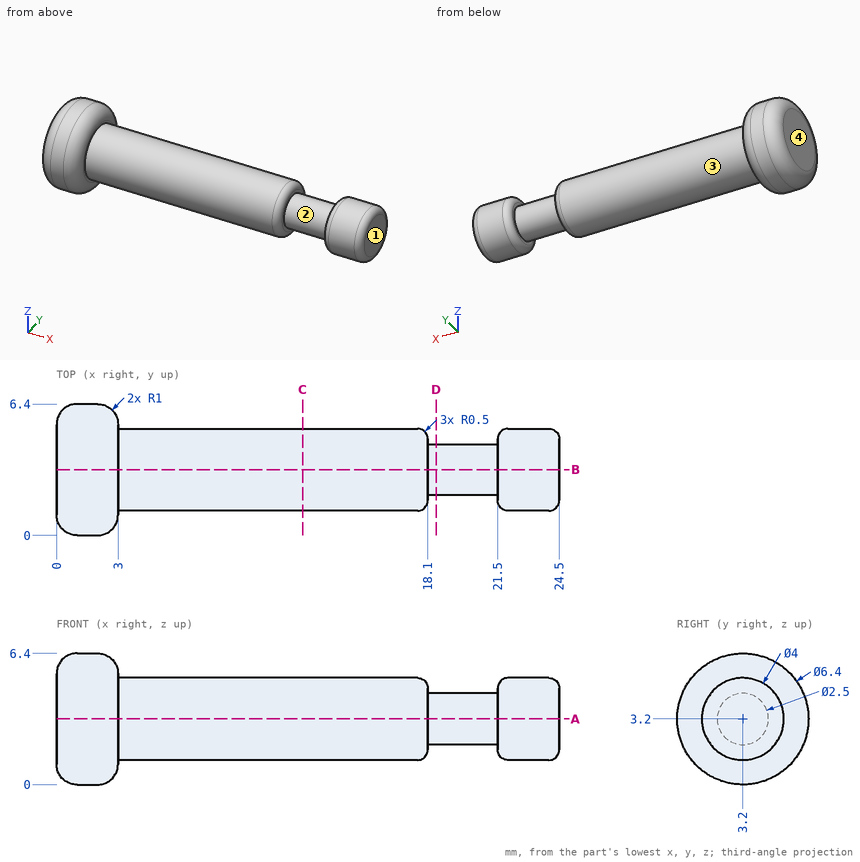
Geometry: see drawing. Coordinates: mm, zero at the bounding-box minimum. Give positions to 0.01 mm unless a question says otherwise; leave off trailing zeros. Order: outer loops, then holes, each group sorted by start corner. A loop starts at its lowest first (then second) coordinate and runs counter-clockwise, first axis right, second up. Notation, with made-up numbers: (86, 39.25) -> (130, 39.25) arc R18 ccw to (130, 64.25) -> close; hole circle Ø7 at (16, -10). An arc over 180 degrees is marked (long way). Write each question's results on one line, items separated by ' | '.
1) Cut plane D-D (x = 18.5). Output: boundary loops of the cut face in (y, z).
Geometry says:
outline: circle Ø2.5 at (3.2, 3.2)
2) Cut plane C-C (x = 12). Output: boundary loops of the cut face in (y, z), and give its area (3 significant figures).
Geometry says:
outline: circle Ø4 at (3.2, 3.2) | area: 12.6 mm²
3) First-contact query: pin 1 Ø3 at (x, y) = (19, 1.5) entering from +Z; pin 2 Ø3 at (x, z) = (17, 4) entering from -Y. Flat tips, straight axial feed; report the tip coordinate or a pass-through.
Geometry says:
pin 1: stops at z = 4.99 | pin 2: stops at y = 1.2
4) Line query: line 1 along X through (y, z) = (2.75, 5.25); line 2 along X through (y, z) = (3.5, 5); line 3 along Z through (x, y) = (15.5, 3). Output: solid intervals per line, ascending.
Geometry says:
line 1: x = 0 to 3 | line 2: x = 0 to 17.98, 21.62 to 24.38 | line 3: z = 1.21 to 5.19
5) Draft query along X for the marked faces 1, 2, 3 and 4. Return one class per face: released by +X, released by -X, zero draft, split by the parting line, or undercut.
Geometry says:
face 1: released by +X | face 2: undercut | face 3: zero draft | face 4: released by -X
6) Cut plane A-A (z = 3.2). Output: boundary loops of the cut face in (x, y), and give its area (3 significant figures).
Geometry says:
outline: (0, 1) arc R1 ccw to (1, 0) -> (2, 0) arc R1 ccw to (3, 1) -> (3, 1.2) -> (17.6, 1.2) arc R0.5 ccw to (18.1, 1.7) -> (18.1, 1.95) -> (21.5, 1.95) -> (21.5, 1.7) arc R0.5 ccw to (22, 1.2) -> (24, 1.2) arc R0.5 ccw to (24.5, 1.7) -> (24.5, 4.7) arc R0.5 ccw to (24, 5.2) -> (22, 5.2) arc R0.5 ccw to (21.5, 4.7) -> (21.5, 4.45) -> (18.1, 4.45) -> (18.1, 4.7) arc R0.5 ccw to (17.6, 5.2) -> (3, 5.2) -> (3, 5.4) arc R1 ccw to (2, 6.4) -> (1, 6.4) arc R1 ccw to (0, 5.4) -> close | area: 98.9 mm²
